```python
from build123d import *

# Parameters (mm, degrees)
BOSS_EXTRUDE1_DEPTH = 19.05
SKETCH6_R           = 19.05
SKETCH6_R_2         = 12.7
BOSS_EXTRUDE3_DEPTH = 127
CUT_EXTRUDE1_REACH  = 321.526
SKETCH7_R           = 12.7
CUT_EXTRUDE2_DEPTH  = 320.525538885


with BuildPart() as part:
    # Sketch1 → Boss-Extrude1 (new body)
    with BuildSketch(Plane(origin=(0, 0, 0), x_dir=(1, 0, 0), z_dir=(0, 1, 0))):
        Polygon((292.1, 76.2), (0, 101.6), (0, 0), (292.1, 0), align=None)
    extrude(amount=BOSS_EXTRUDE1_DEPTH)

    # Sketch6 → Boss-Extrude3 (add)
    # profile 1 of 2: a face of its own
    with BuildSketch(Plane.XY):
        with Locations((114.3, -6.35)):
            Circle(SKETCH6_R)
        with Locations((114.3, -6.35)):
            Circle(SKETCH6_R_2, mode=Mode.SUBTRACT)
    # profile 2 of 2: a face of its own
    with BuildSketch(Plane.XY):
        with Locations((234.95, -6.35)):
            Circle(SKETCH6_R)
        with Locations((234.95, -6.35)):
            Circle(SKETCH6_R_2, mode=Mode.SUBTRACT)
    extrude(amount=-BOSS_EXTRUDE3_DEPTH)

    # Cut-Extrude1: up to this face of the body (flat: up to its plane)
    cut_extrude1_end = Plane(part.part.faces().sort_by_distance((142.169333517, 10.10414021, -89.237449259))[0])
    # Sketch7 → Cut-Extrude1 (cut, up to the picked face)
    with BuildSketch(Plane.XY, mode=Mode.PRIVATE) as cut_extrude1_sk1:
        with Locations((114.3, -6.35)):
            Circle(SKETCH7_R)
    cut_extrude1_tool1 = split(extrude(cut_extrude1_sk1.sketch, amount=-CUT_EXTRUDE1_REACH, mode=Mode.PRIVATE), bisect_by=cut_extrude1_end, keep=Keep.BOTH, mode=Mode.PRIVATE)
    # Sketch7 → Cut-Extrude1 (cut, up to the picked face)
    with BuildSketch(Plane.XY, mode=Mode.PRIVATE) as cut_extrude1_sk2:
        with Locations((234.95, -6.35)):
            Circle(SKETCH7_R)
    cut_extrude1_tool2 = split(extrude(cut_extrude1_sk2.sketch, amount=-CUT_EXTRUDE1_REACH, mode=Mode.PRIVATE), bisect_by=cut_extrude1_end, keep=Keep.BOTH, mode=Mode.PRIVATE)
    add(cut_extrude1_tool1.solids().sort_by(Axis((114.3, -6.35, 0), (0, 0, -1)))[0], mode=Mode.SUBTRACT)
    add(cut_extrude1_tool2.solids().sort_by(Axis((234.95, -6.35, 0), (0, 0, -1)))[0], mode=Mode.SUBTRACT)

    # Sketch8 → Cut-Extrude2 (cut, through all)
    with BuildSketch(Plane.XZ):
        Polygon((132.260512242, -25.4), (0, -25.4), (0, -76.104150603), (132.260512242, -64.603236495), align=None)
        Polygon((216.989487758, -25.4), (132.260512242, -25.4), (132.260512242, -64.603236495), (216.989487758, -57.235499493), align=None)
        Polygon((292.1, -25.4), (216.989487758, -25.4), (216.989487758, -57.235499493), (292.1, -50.704150603), align=None)
    extrude(amount=CUT_EXTRUDE2_DEPTH, mode=Mode.SUBTRACT)


solid = part.part
```
The listing builds one solid part. Answer for the finished solid, in the listing's coordinates (mm). A direction names the side the tool comes from. Round coordinates to 2 decimals unless told otherwise and drop trailing zeros. Loops run counter-clockwise (first coordinate to the right, second up) from the corner with the lowest first, then second, coordinate; pieces in that order, holes last. Notation, with made-up numbers: (7, 73) -> (38, 73) arc R25 cw to (38, 88) -> close; hole circle Ø8 at (2, 8). An arc over 180 degrees is marked (long way). Use one line per item in the form item = value.
1. Find the intervals of material crossed by probe 1 along X at (y, z) = (-6.5, -11.5); probe 2 along Y at (x, z) = (114.3, -76.5); probe 3 along X at (y, z) = (-6.35, -59.5), in increasing order. Write a range as [from, to].
Answer key:
probe_1 = [95.25, 101.6], [127, 133.35], [215.9, 222.25], [247.65, 254]
probe_2 = [-25.4, -19.05], [6.35, 19.05]
probe_3 = [215.9, 222.25], [247.65, 254]
2. The part is cut by section C-C on z = -116. Determine the outline of the cut face in (x, y).
Answer key:
outline = circle Ø38.1 at (114.3, -6.35); circle Ø38.1 at (234.95, -6.35); hole circle Ø25.4 at (114.3, -6.35); hole circle Ø25.4 at (234.95, -6.35)
3. Flat-ended cylindrical pins translate along their axes: pin 1 Ø3 at (y, z) = (-18.5, -67.5) entering from +X; pin 2 Ø10 at (x, z) = (201, -25) entering from -Y; pin 3 Ø12 at (y, z) = (5, -110.5) entering from -X. Find the tip coordinate at first contact, or state that the pin passes through.
Answer key:
pin_1 = 250.74
pin_2 = 0
pin_3 = 96.02
4. The part is cut by section B-B on x = 114.3. Determine the outline of the cut face in (y, z).
Answer key:
outline = (-25.4, -127) -> (-19.05, -127) -> (-19.05, -66.17) -> (-25.4, -66.17) -> close; (-25.4, -25.4) -> (-19.05, -25.4) -> (-19.05, 0) -> (-25.4, 0) -> close; (6.35, -127) -> (12.7, -127) -> (12.7, -91.66) -> (19.05, -91.66) -> (19.05, 0) -> (6.35, 0) -> close
5. For a pull along X with two mould halves and no side action, classify faces 1 (the flat face through (144, 7, 0)), 2 (the cylindrical face through (243.74, -23.25, -90)), 3 (the flat face through (0, 9, -52)) as released by +X, released by -X, zero draft, split by the parting line, or undercut.
Answer key:
face_1 = zero draft
face_2 = undercut
face_3 = released by -X
6. A tool of negligible diameter and unlimited length cuts with its end or side. For faces 4 (the flat face through (292.1, 9, -38)), 5 (the flat face through (235, -21, -25.4)), from which of +Z, -Z, +X, -X, +Y, -Y can it reach the whole face along a straight path? Write none if from no direction.
Answer key:
face_4 = +Z, -Z, +X, +Y, -Y
face_5 = +X, -X, -Y
7. The part is cut by section D-D on y = -3. Give the number of separate pieces and of enclosed holes in the cut face, and give its area (3 significant figures).
Answer key:
separate_pieces = 8
enclosed_holes = 0
area = 2,380 mm²
8. The part is cut by section A-A on z = -39. Determine the outline of the cut face in (x, y).
Answer key:
outline = (0, 0) -> (103.3, 0) arc R12.7 cw to (125.3, 0) -> (223.95, 0) arc R12.7 cw to (245.95, 0) -> (292.1, 0) -> (292.1, 19.05) -> (0, 19.05) -> close
